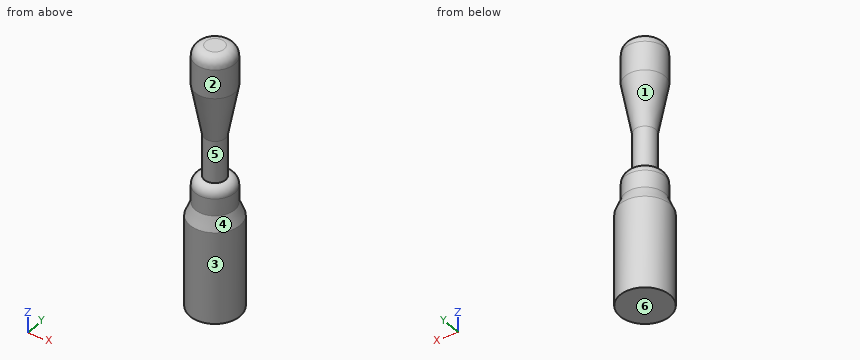
```python
from build123d import *


with BuildPart() as f1:
    # F0 (on Front) → F1 (revolve)
    with BuildSketch(Plane.XZ):
        with BuildLine():
            Line((3.5, 0), (0, 0))
            Line((0, 0), (0, -100))
            Line((0, -100), (9.5, -100))
            Line((9.5, -100), (9.5, -65))
            Line((9.5, -65), (7.5, -60))
            Line((7.5, -60), (7.5, -53.5))
            ThreePointArc((7.5, -53.5), (6.474874, -51.025126), (4, -50))
            Line((4, -50), (4, -34))
            Line((4, -34), (7.5, -15))
            Line((7.5, -15), (7.5, -4))
            ThreePointArc((7.5, -4), (6.328427, -1.171573), (3.5, 0))
        make_face()
    revolve(axis=Axis((0, 0, -50), (0, 0, 1)))


solid = f1.part
```
CAD build for the part. Positions are in the model's coordinates, mm. Face numbers are marked on the shaded views. A direction names the side the tool comes from. Coordinates: 2 decimals unless noted, no trailing zeros. Loops run counter-clockwise (first coordinate to the right, second up) from the corner with the lowest first, then second, coordinate; pieces in that order, holes last. Notation, with made-up numbers: (84, 32.25) - (139, 32.25) arc R13 cw to (139, 40.25) - close; hole circle Ø9 at (3.25, 23.5). An arc over 180 degrees is marked (long way). Return JSON: item names as keys, results as strings.
1. Probe L1, parallel to X at y = -3, z = -21.5; L2, parallel to X at y = 1, z = -33; L3, parallel to Z at x = 5.5, y = -7.5. List the from-to ranges inside material, lowest first. Write a range as from..to.
Result:
{"L1": "x = -5.54..5.54", "L2": "x = -4.06..4.06", "L3": "z = -100..-64.5"}
2. 3-axis set-ups, long thin cutter, end or side, ignore diameter. For the marked faces 1, 2 and 3: which of +Z, -Z, +X, -X, +Y, -Y reach the whole face in a straight line?
Result:
{"face 1": "none", "face 2": "+Z", "face 3": "+Z, -Z"}
3. Drop flat-ended pins along their axis: pin 1 (8 mm diameter, centred on y = 5.5, z = -24, fed in from +X); pin 2 (5 mm diameter, centred on x = -7.5, z = -75.5, fed in from +Y); pin 3 (5 mm diameter, centred on x = 4.5, z = -71, fed in from -Y). Give the stop position or say it passes through.
Result:
{"pin 1": "stops at x = 5.87", "pin 2": "stops at y = 8.08", "pin 3": "stops at y = -9.29"}
4. Mould opens along Z. For the marked faces 4, 5 and 6 say: released by +Z, released by -Z, zero draft, split by the parting line, or undercut.
Result:
{"face 4": "released by +Z", "face 5": "undercut", "face 6": "released by -Z"}
5. Band-saw the part on B-B (z = -12). Give the cut face in (x, y), and give its area (3 significant figures).
Result:
{"outline": "circle Ø15 at (0, 0)", "area": "177 mm2"}
6. Band-saw the part on A-A (z = -77). Give the cut face in (x, y).
Result:
{"outline": "circle Ø19 at (0, 0)"}
